Model file for the job. Use its own axes, mm. A direction names the side the tool comes from. Coordinates: 2 decimals unless noted, no trailing zeros. Write each loop counter-clockwise with the first axis right and the second up, starting at its lowest first coordinate (ties: lowest second). Pieces come first, ordered by that corner, then holes. Notation, with made-up numbers: M 3,-39 L 24,-39 A28 cw 24,-20 Z; hole C 27.25,4.25 d8. An arc over 180 degrees is marked long. Put each result on its own line as item: value. Start each with the question number.
Q1. Drill centre lines: line 1 along Z through (x, y) = (26, -5); line 2 along X through (y, z) = (-11.5, 95); line 3 along Z through (x, y) = (-24, -20.75). Where is each one in solid material? Low to high.
Q2. Drop flat-ended pins along their axis: pin 1 (3 mm diameter, centred on y = -6.5, z = 51, fed in from -X); pin 2 (1.2 mm diameter, centred on x = -24.5, y = -13.5, fed in from +Z); pin 3 (1.5 mm diameter, centred on y = -6, z = 29.5, fed in from +X). Give the stop position or say it passes through.
Q3. Pull direction Z, two halves, no side cores. Call faces 1 (the flat face through (24, -11, 100)), 2 (the flat face through (24, -11, 90)), 3 (the flat face through (0, -22, 52)): pulls with the +Z half, pulls with the -Z half, needs draft (parallel to the pull), parting line crosses it, or undercut.
Q4. Cut at A-A (z = 51.5). Write the cut outline in (x, y).
Q5. Which spindle directions (+Z, -Z, +X, -X, +Y, -Y) get a long thin tool onto all of the face, cutting with end or side? Do faces 4 (the flat face through (-24, -11, 90)), 5 (the flat face through (16, -16, 10)), 6 (the flat face through (17.5, -5, 53)), 7 (the flat face through (-22, -11, 2)), 8 (the flat face through (22, -11, 2)). Say none if no direction does.
Q6. Cut at B-B (y = -8). Give the number of separate pieces and of enclosed holes in the cut face, then the cut area to 3 significant figures.
Autodesk Inventor part; units mm, degrees
ref_plane "YZ Plane" through (0, 0, 0) normal (1, 0, 0) x (0, 1, 0)
ref_plane "XZ Plane" through (0, 0, 0) normal (0, 1, 0) x (-1, 0, 0)
ref_plane "Płaszczyzna konstrukcyjna3" through (0, 0, 35) normal (0, 0, 1) x (1, 0, 0)
ref_plane "Płaszczyzna konstrukcyjna4" through (0, 0, 70) normal (0, 0, 1) x (1, 0, 0)
ref_plane "Płaszczyzna konstrukcyjna5" through (0, 0, 105) normal (0, 0, 1) x (1, 0, 0)
sketch "Szkic7" plane through (0, 0, 0) normal (0, 0, 1) x (1, 0, 0)
  circle A0 centre (0, 0) radius 19
  dimension "d41" = 38
sketch "Szkic9" plane through (0, 0, 35) normal (0, 0, 1) x (1, 0, 0)
  line L0 (16.5, 10.25) -> (-16.5, 10.25)
  line L1 (-16.5, 10.25) -> (-16.5, -10.25)
  line L2 (-16.5, -10.25) -> (16.5, -10.25)
  line L3 (16.5, -10.25) -> (16.5, 10.25)
  line L4 (16.5, 10.25) -> (-16.5, -10.25) construction
  line L5 (-16.5, 10.25) -> (16.5, -10.25) construction
  point P0 (0, 0)
  dimension "d42" = 33
  dimension "d43" = 20.5
sketch "Szkic10" plane through (0, 0, 70) normal (0, 0, 1) x (1, 0, 0)
  line L0 (16.5, 10.25) -> (-16.5, 10.25)
  line L1 (-16.5, 10.25) -> (-16.5, -10.25)
  line L2 (-16.5, -10.25) -> (16.5, -10.25)
  line L3 (16.5, -10.25) -> (16.5, 10.25)
  point P0 (0, 0)
sketch "Szkic11" plane through (0, 0, 105) normal (0, 0, 1) x (1, 0, 0)
  line L0 (20, -20) -> (-20, -20)
  line L1 (-20, -20) -> (-20, 20)
  line L2 (-20, 20) -> (20, 20)
  line L3 (20, 20) -> (20, -20)
  line L4 (20, -20) -> (-20, 20) construction
  line L5 (-20, -20) -> (20, 20) construction
  point P0 (0, 0)
  dimension "d44" = 40
  dimension "d45" = 40
sketch "Szkic12" plane through (0, 0, 0) normal (0, 0, 1) x (1, 0, 0)
  line L0 (-22, -22) -> (22, -22)
  line L1 (22, -22) -> (22, 22)
  line L2 (22, 22) -> (-22, 22)
  line L3 (-22, 22) -> (-22, -22)
  line L4 (-22, -22) -> (22, 22) construction
  line L5 (22, -22) -> (-22, 22) construction
  point P0 (0, 0)
  dimension "d46" = 44
  dimension "d47" = 44
extrude "Wyciągnięcie proste1" add sketch "Szkic12" along normal blind 105
extrude "Wyciągnięcie proste2" cut sketch "Szkic9" along normal blind 35
loft "Wyciągnięcie złożone1" cut profiles "Szkic7" section 2 edges at (-16.5, 0, 35) (0, -10.25, 35) (16.5, 0, 35) (0, 10.25, 35)
loft "Wyciągnięcie złożone2" cut profiles "Szkic11" section 2 edges at (-16.5, 0, 70) (0, 10.25, 70) (16.5, 0, 70) (0, -10.25, 70)
sketch "Szkic13" plane through (0, 0, 70) normal (0, 0, 1) x (1, 0, 0)
  line L0 (-17.5, -10.25) -> (17.5, -10.25)
  line L1 (17.5, -10.25) -> (17.5, 10.25)
  line L2 (17.5, 10.25) -> (-17.5, 10.25)
  line L3 (-17.5, 10.25) -> (-17.5, -10.25)
  line L4 (-17.5, -10.25) -> (17.5, 10.25) construction
  line L5 (17.5, -10.25) -> (-17.5, 10.25) construction
  point P0 (0, 0)
  dimension "d60" = 35
  dimension "d61" = 20.5
extrude "Wyciągnięcie proste3" cut sketch "Szkic13" against normal blind 35
sketch "Szkic14" plane through (-22, 22, 0) normal (0, 1, 0) x (1, 0, 0)
  point P0 (22, 0)
sketch "Szkic15" plane through (-16.2734, 10.25, 35) normal (0, -1, 0) x (1, 0, 0)
  line L0 (32.5467, 0) -> (0, 0) construction
  line L1 (16.2734, 0) -> (16.2734, -12) construction
  circle A0 centre (16.2734, -12) radius 4
  point P0 (16.2734, -35)
  dimension "d64" = 12
  dimension "d65" = 8
extrude "Wyciągnięcie proste4" cut sketch "Szkic15" against normal through all
sketch "Szkic16" plane through (0, 0, 0) normal (0, 0, -1) x (-1, 0, 0)
  line L0 (-16, -16) -> (16, -16) construction
  line L1 (16, -16) -> (16, 16) construction
  line L2 (16, 16) -> (-16, 16) construction
  line L3 (-16, 16) -> (-16, -16) construction
  line L4 (-16, -16) -> (16, 16) construction
  line L5 (16, -16) -> (-16, 16) construction
  circle A0 centre (-16, 16) radius 1.5
  circle A1 centre (-16, -16) radius 1.5
  circle A2 centre (16, -16) radius 1.5
  circle A3 centre (16, 16) radius 1.5
  point P0 (0, 0)
  dimension "d68" = 32
  dimension "d69" = 32
  dimension "d70" = 3
extrude "Wyciągnięcie proste5" cut sketch "Szkic16" against normal blind 10
sketch "Szkic17" plane through (0, 0, 0) normal (0, 1, 0) x (-1, 0, 0)
  line L0 (-35.497, 120.9522) -> (40.1676, 120.9522)
  line L1 (40.1676, 120.9522) -> (40.1676, -13.5628)
  line L2 (40.1676, -13.5628) -> (-35.497, -13.5628)
  line L3 (-35.497, -13.5628) -> (-35.497, 120.9522)
  point P0 (0, 0)
sketch "Szkic18" plane through (-22, 22, 0) normal (0, 1, 0) x (1, 0, 0)
  point P0 (22, 0)
sketch "Szkic19" plane through (-22, 22, 0) normal (0, 1, 0) x (1, 0, 0)
  line L0 (44, 0) -> (44, -105)
  line L1 (44, -105) -> (44, -95) construction
  line L2 (44, -95) -> (48, -95) construction
  arc A0 (48, -100) -> (48, -90) centre (48, -95) ccw
  line L3 (48, -100) -> (44, -100)
  line L4 (48, -90) -> (44, -90)
  line L5 (44, -100) -> (44, -90)
  line L6 (22, -110.411) -> (22, 7.1772) construction
  line L7 (-9.1147, -52.5) -> (56.3126, -52.5) construction
  line L8 (44, -10) -> (48, -10) construction
  arc A1 (48, -15) -> (48, -5) centre (48, -10) ccw
  line L9 (48, -5) -> (44, -5)
  line L10 (48, -15) -> (44, -15)
  line L11 (44, -5) -> (44, -15)
  line L12 (0, 0) -> (0, -105)
  line L13 (0, -105) -> (0, -95) construction
  line L14 (0, -95) -> (-4, -95) construction
  arc A2 (-4, -90) -> (-4, -100) centre (-4, -95) ccw
  line L15 (-4, -100) -> (0, -100)
  line L16 (-4, -90) -> (0, -90)
  line L17 (0, -100) -> (0, -90)
  line L18 (0, -10) -> (-4, -10) construction
  arc A3 (-4, -5) -> (-4, -15) centre (-4, -10) ccw
  line L19 (-4, -5) -> (0, -5)
  line L20 (-4, -15) -> (0, -15)
  line L21 (0, -5) -> (0, -15)
  point P0 (22, 0)
  dimension "d73" = 10
  dimension "d74" = 4
  dimension "d75" = 10
extrude "Wyciągnięcie proste6" add sketch "Szkic19" against normal up to surface (44 mm away)
sketch "Szkic20" plane through (-22, 22, 0) normal (0, 1, 0) x (1, 0, 0)
  arc A0 (48, -15) -> (48, -5) centre (48, -10) ccw
  arc A1 (-4, -5) -> (-4, -15) centre (-4, -10) ccw
  arc A2 (-4, -90) -> (-4, -100) centre (-4, -95) ccw
  arc A3 (48, -100) -> (48, -90) centre (48, -95) ccw
  point P0 (22, 0)
hole "Otwór1" at (26, 22, 10) at (-26, 22, 10) at (26, 22, 95) at (-26, 22, 95) direction (0, -1, 0) diameter 3 end through all counterbore diameter 5 counterbore depth 2
extrude "Wyciągnięcie proste7" cut sketch "Szkic17" along normal up to surface (22 mm away)
properties part number "heater_case_bottom"
Computed values:
1. line 1: 5 to 8.5, 11.5 to 15, 90 to 93.5, 96.5 to 100
1. line 2: -31 to -27.5, -24.5 to -19, 19 to 24.5, 27.5 to 31
1. line 3: 5 to 15, 90 to 100
2. pin 1: x = -22
2. pin 2: z = 100
2. pin 3: x = 22
3. face 1: pulls with the +Z half
3. face 2: undercut
3. face 3: needs draft
4. outline: M -22,-22 L 22,-22 L 22,0 L 17.5,0 L 17.5,-10.25 L -17.5,-10.25 L -17.5,0 L -22,0 Z
5. face 4: -X, +Y, -Y
5. face 5: -Z
5. face 6: +Y
5. face 7: -Z, -X, +Y, -Y
5. face 8: -Z, +X, +Y, -Y
6. separate pieces: 2
6. enclosed holes: 4
6. area: 1,230 mm2
